Source: CAD feature listing. Evaluate the final solid. Frame: model axes, mm. Face numbers are marked on the shaded views. Round coordinates to 2 decimals unless told otherwise and drop trailing zeros. Order: outer loops, then holes, each group sorted by start corner. A loop starts at its lowest first (then second) coordinate and runs counter-clockwise, first axis right, second up. Notation, with made-up numbers: M -19.75,46.5 L 14.25,46.5 A18 ccw 14.25,60.5 Z; hole C 34,-17.75 d9. An arc over 180 degrees is marked long. Answer in a Markdown table with one row per item. Add a question column.
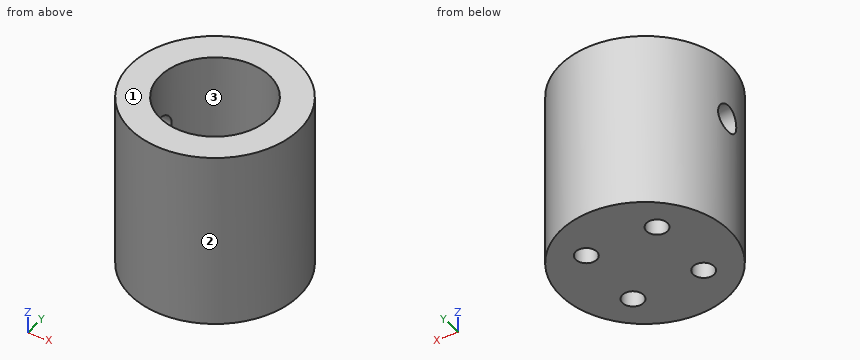
```python
from build123d import *

# Parameters (mm, degrees)
SKETCH_1_R          = 10
EXTRUDE_1_DEPTH     = 21
SKETCH_2_R          = 6.5
CUT_EXTRUDE_1_DEPTH = 15
M4X0_71_D           = 3.3
M4X0_71_DEPTH       = 5
M4X0_71_TIP         = 0.991420021
M3X0_51_D           = 2.5
M3X0_51_DEPTH       = 6


with BuildPart() as part:
    # Эскиз1 → Бобышка-Вытянуть1 (new body)
    with BuildSketch(Plane.XY):
        with Locations(Location((0, 0, 0), (0, 0, 180))):
            Circle(SKETCH_1_R)
    extrude(amount=EXTRUDE_1_DEPTH)

    # Эскиз2 → Вырез-Вытянуть1 (cut)
    with BuildSketch(Plane.XY.offset(21)):
        Circle(SKETCH_2_R)
    extrude(amount=-CUT_EXTRUDE_1_DEPTH, mode=Mode.SUBTRACT)

    # Отверстие обработанное метчиком M4x0.71
    with Locations(Plane(origin=(-10, 0, 0), x_dir=(0, 0, -1), z_dir=(-1, 0, 0))):
        with Locations((-14, 0)):
            Hole(M4X0_71_D / 2, depth=M4X0_71_DEPTH)
            with Locations((0, 0, -(M4X0_71_DEPTH + M4X0_71_TIP / 2))):  # 118° drill point
                Cone(0, M4X0_71_D / 2, M4X0_71_TIP, mode=Mode.SUBTRACT)

    # Отверстие обработанное метчиком M3x0.51
    with Locations(Plane(origin=(0, 0, 0), x_dir=(-1, 0, 0), z_dir=(0, 0, -1))):
        with Locations((-4.242640687, 4.242640687), (4.242640687, 4.242640687), (4.242640687, -4.242640687), (-4.242640687, -4.242640687)):
            Hole(M3X0_51_D / 2, depth=M3X0_51_DEPTH)


solid = part.part
```
(1) Line query: line 1 (Y direction, x = 0, z = 10); line 2 (X direction, y = 1, z = 18); line 3 (Y direction, x = 6, z = 8). Output: solid intervals per line, ascending. Write a range as from..to.
(2) Cut plane C-C (z = 7.5). Return loops of the section in (x, y), and give its area (3 significant figures).
(3) Pin query (flat end, axial travel): pin 1 (6 mm diameter, centred on x = 2.5, z = 15.5, fed in from +Y); pin 2 (1.5 mm diameter, centred on x = 4.5, y = 4.5, fed in from -Z); pin 3 (6.5 mm diameter, centred on x = 2.5, y = 0.5, fed in from +Z); pin 4 (2 mm diameter, centred on x = -7, z = 3.5, fed in from -Y). Return the tip coordinate at first contact, or that it passes through.
(4) Cut plane B-B (x = 0). Return loops of the section in (y, z).
(5) Draft query along Y for the marked faces 1, 2 and 3. Return one class per face: +Y half, -Y half, draft (parallel to the pull), parting line (faces both ways), or undercut.
(6) Cut plane D-D (x = -7.75). Return loops of the section in (y, z).
(7) Cut plane A-A (y = 0). Return loops of the section in (x, z).
Answer list:
| question | item | result |
|---|---|---|
| 1 | line 1 | -10..-6.5, 6.5..10 |
| 1 | line 2 | -9.95..-6.42, 6.42..9.95 |
| 1 | line 3 | -8..-2.5, 2.5..8 |
| 2 | outline | C 0,0 d20; hole C 0,0 d13 |
| 2 | area | 181 mm² |
| 3 | pin 1 | y = 10 |
| 3 | pin 2 | z = 6 |
| 3 | pin 3 | z = 6 |
| 3 | pin 4 | y = -8 |
| 4 | outline | M -10,0 L 10,0 L 10,21 L 6.5,21 L 6.5,6 L -6.5,6 L -6.5,21 L -10,21 Z |
| 5 | face 1 | draft |
| 5 | face 2 | parting line |
| 5 | face 3 | undercut |
| 6 | outline | M -6.32,0 L 6.32,0 L 6.32,21 L -6.32,21 Z; hole C 0,14 d3.3 |
| 7 | outline | M -10,0 L 10,0 L 10,21 L 6.5,21 L 6.5,6 L -6.5,6 L -6.5,12.35 L -10,12.35 Z; M -10,15.65 L -6.5,15.65 L -6.5,21 L -10,21 Z |
